Work out the finished part from the listing and answer in its coordinate system (mm). Give positions to 0.01 mm unless a question says otherwise; leave off trailing zeros. Loops run counter-clockwise (first coordinate to the right, second up) from the corner with the lowest first, then second, coordinate; pieces in that order, holes last. Notation, with made-up numbers: M 43,70 L 64,70 A20 ccw 64,83 Z; hole C -35.5,-7 d5. An arc over 180 degrees is marked long. Use a Markdown table: item, result.
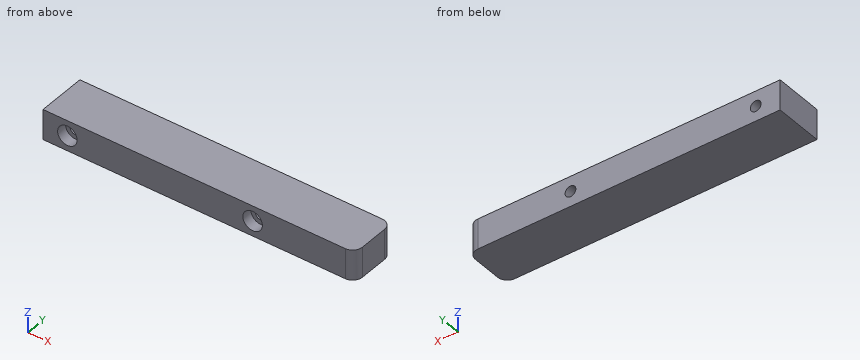
```python
from build123d import *

# Parameters (mm, degrees)
SKETCH1_W                                           = 15.5
SKETCH1_H                                           = 25
BOSS_EXTRUDE1_DEPTH                                 = 80
CBORE_FOR_M5_HEX_SOCKET_HEAD_CAP_SCREW1_D           = 5.5
CBORE_FOR_M5_HEX_SOCKET_HEAD_CAP_SCREW1_CBORE_D     = 10
CBORE_FOR_M5_HEX_SOCKET_HEAD_CAP_SCREW1_CBORE_DEPTH = 5.4
FILLET1_R                                           = 5
FILLET2_R                                           = 5


with BuildPart() as part:
    # Sketch1 → Boss-Extrude1 (new body, symmetric)
    with BuildSketch(Plane(origin=(0, 0, 0), x_dir=(0, 0, -1), z_dir=(1, 0, 0))):
        Rectangle(SKETCH1_W, SKETCH1_H)
    extrude(amount=BOSS_EXTRUDE1_DEPTH, both=True)

    # CBORE for M5 Hex Socket Head Cap Screw1 (through all)
    with Locations(Plane(origin=(0, -12.5, 0), x_dir=(-1, 0, 0), z_dir=(0, -1, 0))):
        with Locations((-27.5, 0), (67.5, 0)):
            CounterBoreHole(CBORE_FOR_M5_HEX_SOCKET_HEAD_CAP_SCREW1_D / 2, CBORE_FOR_M5_HEX_SOCKET_HEAD_CAP_SCREW1_CBORE_D / 2, CBORE_FOR_M5_HEX_SOCKET_HEAD_CAP_SCREW1_CBORE_DEPTH)

    # Fillet1
    fillet1_edges = [part.edges().sort_by_distance(p)[0] for p in [
        (80, -12.5, 0),
    ]]
    fillet(fillet1_edges, radius=FILLET1_R)

    # Fillet2
    fillet2_edges = [part.edges().sort_by_distance(p)[0] for p in [
        (80, 12.5, 0),
    ]]
    fillet(fillet2_edges, radius=FILLET2_R)


solid = part.part
```
(1) Consider probe 1 along Z at (x, y) = (27.5, -10.95); probe 2 along X at (y, z) = (7.25, -1); probe 3 along X at (y, z) = (-10, 1.5). Determine where each line is inside the solid, lowest interval first. Write a range as [from, to].
Entries:
| item | result |
|---|---|
| probe 1 | z = [-7.75, -5], [5, 7.75] |
| probe 2 | x = [-80, -70.06], [-64.94, 24.94], [30.06, 80] |
| probe 3 | x = [-80, -72.27], [-62.73, 22.73], [32.27, 79.33] |
(2) A cutting plane is placed at A-A (x = 27.5). Write down the section's boundary in (y, z).
Entries:
| item | result |
|---|---|
| outline | M -12.5,-7.75 L 12.5,-7.75 L 12.5,-2.75 L -7.1,-2.75 L -7.1,-5 L -12.5,-5 Z; M -12.5,5 L -7.1,5 L -7.1,2.75 L 12.5,2.75 L 12.5,7.75 L -12.5,7.75 Z |
(3) A cutting plane is placed at C-C (y = 1.75). Write down the section's boundary in (x, z), and give its area (3 significant figures).
Entries:
| item | result |
|---|---|
| outline | M -80,-7.75 L 80,-7.75 L 80,7.75 L -80,7.75 Z; hole C -67.5,0 d5.5; hole C 27.5,0 d5.5 |
| area | 2,430 mm² |
(4) A cutting plane is placed at B-B (z = 0). Write down the section's boundary in (x, y), and give its area (3 significant figures).
Entries:
| item | result |
|---|---|
| outline | M -80,-12.5 L -72.5,-12.5 L -72.5,-7.1 L -70.25,-7.1 L -70.25,12.5 L -80,12.5 Z; M -64.75,-7.1 L -62.5,-7.1 L -62.5,-12.5 L 22.5,-12.5 L 22.5,-7.1 L 24.75,-7.1 L 24.75,12.5 L -64.75,12.5 Z; M 30.25,-7.1 L 32.5,-7.1 L 32.5,-12.5 L 75,-12.5 A5 ccw 80,-7.5 L 80,7.5 A5 ccw 75,12.5 L 30.25,12.5 Z |
| area | 3,670 mm² |
(5) Given P1, Ø5, axis at x = 27.5, z = 0, coming from the -Y side; P2, Ø3, axis at x = 27, z = 2, coming from the -Y side, each flat-ended and moving along its own axis, determine where each tip first touches the part or whether it passes through.
Entries:
| item | result |
|---|---|
| P1 | passes through |
| P2 | stops at y = -7.1 |
